Verification items for the finished model (mm, model axes). A direction names the side the tool comes from. Give positions to 0.01 mm unless a question says otherwise; leave off trailing zeros. Write each question's results on one line, items separated by ' | '. Start each with the question number.
1. Set-up check for faces 1 (the face through (14.92, 1.55, 49.3)), 2 (the face through (-2.17, -9.76, -1.48)): record each of +Z, -Z, +X, -X, +Y, -Y from which the full face is reachable in a straight line by a thin tool's end or side.
2. Mould release check, pull along X, two halves, no side actions. Record for faces 3 (the face through (6.09, -13.71, 49.3)), 4 (the face through (11.28, -6.46, 50.7)), 5 (the face through (-2.17, -9.76, 101.48)): +X half, -X half, draft (parallel to the pull), parting line (faces both ways), or undercut.
3. Material ranges on L1, parallel to Y at x = 0, z = 101.8; L2, parallel to X at y = 4, z = 84.5; L3, parallel to Z at x = 6, y = -3, recorded low to high. Write a range as from..to.
4. Depth check by flat-ended pin: pin 1 Ø2.5 at (x, y) = (5.3, -5.3) entering from -Z; pin 2 Ø1.6 at (x, y) = (-5, 5.5) entering from +Z; pin 3 Ø1.6 at (x, y) = (0, 7.5) entering from +Z. Enter the tip coordinate at first touch or a pass-through.
from build123d import *

# Parameters (mm, degrees)
SKETCH1_R           = 15
BOSS_EXTRUDE1_DEPTH = 100
SKETCH2_R           = 2.5
BOSS_EXTRUDE3_DEPTH = 15
SKETCH4_R           = 10
SKETCH4_R_2         = 2.5
BOSS_EXTRUDE4_DEPTH = 3
SKETCH7_R           = 1
CUT_EXTRUDE1_DEPTH  = 3
SKETCH8_R           = 2
CUT_EXTRUDE2_DEPTH  = 116


with BuildPart() as part:
    # Sketch1 → Boss-Extrude1 (new body)
    with BuildSketch(Plane.XY):
        Circle(SKETCH1_R)
    extrude(amount=BOSS_EXTRUDE1_DEPTH)

    # Sketch2 → Boss-Extrude3 (add)
    with BuildSketch(Plane.XY.offset(100)):
        Circle(SKETCH2_R)
    boss_extrude3 = extrude(amount=BOSS_EXTRUDE3_DEPTH)

    # Sketch4 → Boss-Extrude4 (add)
    with BuildSketch(Plane.XY.offset(100)):
        Circle(SKETCH4_R)
        Circle(SKETCH4_R_2, mode=Mode.SUBTRACT)
    boss_extrude4 = extrude(amount=BOSS_EXTRUDE4_DEPTH)

    # Mirror1: Boss-Extrude3, Boss-Extrude4 across plane
    add(boss_extrude3.mirror(Plane.XY.offset(50)))
    add(boss_extrude4.mirror(Plane.XY.offset(50)))

    # Sketch7 → Cut-Extrude1 (cut)
    with BuildSketch(Plane.XY.offset(103)):
        with Locations((0, 7.5)):
            Circle(SKETCH7_R)
        with Locations((5.303300859, 5.303300859)):
            Circle(SKETCH7_R)
        with Locations((7.5, 0)):
            Circle(SKETCH7_R)
        with Locations((5.303300859, -5.303300859)):
            Circle(SKETCH7_R)
        with Locations((0, -7.5)):
            Circle(SKETCH7_R)
        with Locations((-5.303300859, -5.303300859)):
            Circle(SKETCH7_R)
        with Locations((-7.5, 0)):
            Circle(SKETCH7_R)
        with Locations((-5.303300859, 5.303300859)):
            Circle(SKETCH7_R)
    extrude(amount=-CUT_EXTRUDE1_DEPTH, mode=Mode.SUBTRACT)

    # Sketch8 → Cut-Extrude2 (cut, through all)
    with BuildSketch(Plane.XY.offset(100)):
        with Locations((0, 15)):
            Circle(SKETCH8_R)
        with Locations((6.101049646, 13.703181865)):
            Circle(SKETCH8_R)
        with Locations((11.147172382, 10.036959095)):
            Circle(SKETCH8_R)
        with Locations((14.265847744, 4.635254916)):
            Circle(SKETCH8_R)
        with Locations((14.917828431, -1.567926949)):
            Circle(SKETCH8_R)
        with Locations((12.990381057, -7.5)):
            Circle(SKETCH8_R)
        with Locations((8.816778784, -12.135254916)):
            Circle(SKETCH8_R)
        with Locations((3.118675362, -14.672214011)):
            Circle(SKETCH8_R)
        with Locations((-3.118675362, -14.672214011)):
            Circle(SKETCH8_R)
        with Locations((-8.816778784, -12.135254916)):
            Circle(SKETCH8_R)
        with Locations((-12.990381057, -7.5)):
            Circle(SKETCH8_R)
        with Locations((-14.917828431, -1.567926949)):
            Circle(SKETCH8_R)
        with Locations((-14.265847744, 4.635254916)):
            Circle(SKETCH8_R)
        with Locations((-11.147172382, 10.036959095)):
            Circle(SKETCH8_R)
        with Locations((-6.101049646, 13.703181865)):
            Circle(SKETCH8_R)
    extrude(amount=-CUT_EXTRUDE2_DEPTH, mode=Mode.SUBTRACT)


solid = part.part
Results below:
1) face 1: +Z, -Z, +X, +Y | face 2: -Z
2) face 3: +X half | face 4: undercut | face 5: parting line
3) L1: y = -10..-8.5, -6.5..6.5, 8.5..10 | L2: x = -12.37..12.37 | L3: z = -3..103
4) pin 1: stops at z = -3 | pin 2: stops at z = 103 | pin 3: stops at z = 100
